from build123d import *

# Parameters (mm, degrees)
F0_R      = 2.15265
F1_DEPTH  = 66.04
F2_R      = 1.7272
F2_R_2    = 2.15265
F3_DEPTH  = 34.6075
F4_R      = 2.15265
F5_DEPTH  = 38.4175
F7_DEPTH  = 66.04
F9_W      = 23.8125
F9_H      = 9.525
F9_H_2    = 36.3855
F9_H_3    = 10.6045
F10_DEPTH = 27.6225


with BuildPart() as f1:
    # F0 (on Top) → F1 (new body)
    with BuildSketch(Plane.XY):
        Polygon((0, 34.6075), (0, 0), (38.4175, 0), (38.4175, 10.795), (38.4175, 34.6075), (10.795, 34.6075), align=None)
        with Locations((5.3975, 5.3975)):
            Circle(F0_R, mode=Mode.SUBTRACT)
        with Locations((33.02, 5.3975)):
            Circle(F0_R, mode=Mode.SUBTRACT)
        with Locations((5.3975, 29.21)):
            Circle(F0_R, mode=Mode.SUBTRACT)
    extrude(amount=F1_DEPTH)

    # F2 (on face) → F3 (cut, through all)
    with BuildSketch(Plane.XZ):
        with Locations((24.13, 60.198)):
            Circle(F2_R)
        with Locations((24.13, 36.322)):
            Circle(F2_R)
        with Locations((24.13, 4.7625)):
            Circle(F2_R_2)
    extrude(amount=-F3_DEPTH, mode=Mode.SUBTRACT)

    # F4 (on face) → F5 (cut, through all)
    with BuildSketch(Plane(origin=(0, 0, 0), x_dir=(0, -1, 0), z_dir=(-1, 0, 0))):
        with Locations((-20.32, 61.2775)):
            Circle(F4_R)
        with Locations((-20.32, 4.7625)):
            Circle(F4_R)
    extrude(amount=-F5_DEPTH, mode=Mode.SUBTRACT)

    # F6 (on face) → F7 (cut, through all)
    with BuildSketch(Plane.XY.offset(66.04)):
        Polygon((38.4175, 10.795), (38.4175, 34.6075), (10.795, 34.6075), align=None)
    extrude(amount=-F7_DEPTH, mode=Mode.SUBTRACT)

    # F9 (on face) → F10 (cut, through all)
    with BuildSketch(Plane.YZ.offset(38.4175)):
        with Locations((22.70125, 4.7625)):
            Rectangle(F9_W, F9_H)
        with Locations((22.70125, 32.48025)):
            Rectangle(F9_W, F9_H_2)
        with Locations((22.70125, 60.73775)):
            Rectangle(F9_W, F9_H_3)
    extrude(amount=-F10_DEPTH, mode=Mode.SUBTRACT)


solid = f1.part
Build history of the part. All positions in model axes, mm. A direction names the side the tool comes from. Coordinates: 2 decimals unless noted, no trailing zeros. Write each loop counter-clockwise with the first axis right and the second up, starting at its lowest first coordinate (ties: lowest second). Pieces come first, ordered by that corner, then holes.
(1) Cut at D-D on z = 50. List the corners of the cut face in (x, y) (1 decimal), and give its area (3 significant figures).
(2) Cut at B-B on x = 4. List the corners of the cut face in (y, z).
(3) Drill centre lines: line 1 (Z direction, x = 3.25, y = 20.32); line 2 (Z direction, x = 24, y = 4); line 3 (X direction, y = 4, z = 30). Where is each one in solid material? Low to high.
(4) Cut at C-C on y = 20.32. List the corners of the cut face in (x, z) (1 decimal), and give its area (3 significant figures).
(5) Mould opens along X. For faces 6 (the cylindrical face through (5.32, 20.6, 63.41)), 7 (the cylindrical face through (5.117, 31.344, 32.558)), 8 (the cylindrical face through (25.725, 5.322, 59.536)), 9 (the flat face through (38.418, 5, 33)) say: pulls with the +X half, pulls with the -X half, needs draft (parallel to the pull), parting line crosses it, or undercut.
(6) 3-axis set-ups, long thin cutter, end or side, ignore diameter. For faces 1 (the cylindrical face through (26.183, 5.322, 5.409)), 2 (the flat face through (19, 17, 55.436)), 3 (the cylindrical face through (5.32, 22.47, 4.86)), 4 (the flat face through (10.795, 23, 33)), 5 (the flat face through (19, 17, 9.525)): which of +Z, -Z, +X, -X, +Y, -Y reach the whole face in a straight line?
(7) Cut at A-A on z = 5.5. List the corners of the cut face in (x, y) (1 decimal), and give its area (3 significant figures).
(8) Pin check, flat tips, straight feed: pin 1 Ø3 at (y, z) = (20, 53) entering from -X; pin 2 Ø5.5 at (x, z) = (28, 59) entering from +Y (3 decimals); pin 3 Ø4 at (x, z) = (27, 55) entering from +Y; pin 4 Ø12 at (x, y) = (24, 23) entering from +Z. Stop position of each tip, or through.
Working result:
1. outline: (0, 0) - (38.4, 0) - (38.4, 10.8) - (10.8, 10.8) - (10.8, 34.6) - (0, 34.6) - close; hole circle Ø4.3 at (5.4, 5.4); hole circle Ø4.3 at (5.4, 29.2); hole circle Ø4.3 at (33, 5.4)
1. area: 628 mm2
2. outline: (0, 0) - (3.76, 0) - (3.76, 66.04) - (0, 66.04) - close; (7.03, 0) - (27.57, 0) - (27.57, 66.04) - (7.03, 66.04) - close; (30.85, 0) - (34.61, 0) - (34.61, 66.04) - (30.85, 66.04) - close; hole circle Ø4.31 at (20.32, 4.76); hole circle Ø4.31 at (20.32, 61.28)
3. line 1: z = 0 to 2.61, 6.92 to 59.12, 63.43 to 66.04
3. line 2: z = 0 to 2.61, 6.91 to 34.6, 38.04 to 58.48, 61.92 to 66.04
3. line 3: x = 0 to 3.76, 7.03 to 31.38, 34.66 to 38.42
4. outline: (0, 0) - (10.8, 0) - (10.8, 2.6) - (0, 2.6) - close; (0, 6.9) - (10.8, 6.9) - (10.8, 9.5) - (27.4, 9.5) - (27.4, 14.3) - (10.8, 14.3) - (10.8, 50.7) - (27.4, 50.7) - (27.4, 55.4) - (10.8, 55.4) - (10.8, 59.1) - (0, 59.1) - close; (0, 63.4) - (10.8, 63.4) - (10.8, 66) - (0, 66) - close
4. area: 778 mm2
5. face 6: needs draft
5. face 7: undercut
5. face 8: undercut
5. face 9: pulls with the +X half
6. face 1: +Y, -Y
6. face 2: +Z, +X, +Y
6. face 3: +X, -X
6. face 4: +X, +Y
6. face 5: -Z, +X, +Y
7. outline: (0, 0) - (22.1, 0) - (22.1, 10.8) - (10.8, 10.8) - (10.8, 18.3) - (0, 18.3) - close; (0, 22.3) - (10.8, 22.3) - (10.8, 34.6) - (0, 34.6) - close; (26.2, 0) - (38.4, 0) - (38.4, 10.8) - (26.2, 10.8) - close; hole circle Ø4.3 at (5.4, 5.4); hole circle Ø4.3 at (5.4, 29.2); hole circle Ø4.3 at (33, 5.4)
7. area: 541 mm2
8. pin 1: stops at x = 0
8. pin 2: stops at y = 10.795
8. pin 3: stops at y = 22.36
8. pin 4: stops at z = 55.44
